Can you work these out from the model? Positions are in its coordinate system, mm. A direction names the side the tool comes from. Coordinates: 2 decimals unless noted, no trailing zeros. Order: outer loops, then holes, each group sorted by start corner. A loop starts at its lowest first (then second) coordinate and runs counter-clockwise, first axis right, second up.
```python
from build123d import *

# Parameters (mm, degrees)
F0_R           = 4.1275
F1_DEPTH       = 15.875
F3_D           = 8.255
F3_DEPTH       = 25.4
F3_CSINK_D     = 15.24
F3_CSINK_ANGLE = 90
F4_R           = 4.7625
F5_DEPTH       = 19.05


with BuildPart() as f1:
    # F0 (on Front) → F1 (new body)
    with BuildSketch(Plane.XZ):
        with BuildLine():
            ThreePointArc((0, -34.925), (-19.48747, -28.982653), (-32.343511, -13.177743))
            ThreePointArc((-32.343511, -13.177743), (-39.844625, -12.301191), (-45.625986, -17.160297))
            Line((-45.625986, -17.160297), (-72.23125, -70.2945))
            Line((-72.23125, -70.2945), (-72.23125, -89.3445))
            Line((-72.23125, -89.3445), (-56.35625, -89.3445))
            Line((-56.35625, -89.3445), (-56.35625, -86.1695))
            ThreePointArc((-56.35625, -86.1695), (-56.424398, -84.209267), (-56.35625, -82.249034))
            ThreePointArc((-56.35625, -82.249034), (-47.874791, -63.97181), (-29.36658, -56.007))
            ThreePointArc((-29.36658, -56.007), (-28.197928, -55.982797), (-27.029276, -56.007))
            Line((-27.029276, -56.007), (0, -56.007))
            Line((0, -56.007), (0, -34.925))
        make_face()
        with Locations((-37.109015, -21.4249)):
            Circle(F0_R, mode=Mode.SUBTRACT)
        with BuildLine():
            ThreePointArc((32.343511, -13.177743), (19.48747, -28.982653), (0, -34.925))
            Line((0, -34.925), (0, -56.007))
            Line((0, -56.007), (27.029276, -56.007))
            ThreePointArc((27.029276, -56.007), (28.197928, -55.982797), (29.36658, -56.007))
            ThreePointArc((29.36658, -56.007), (47.874791, -63.97181), (56.35625, -82.249034))
            ThreePointArc((56.35625, -82.249034), (56.424398, -84.209267), (56.35625, -86.1695))
            Line((56.35625, -86.1695), (56.35625, -89.3445))
            Line((56.35625, -89.3445), (72.23125, -89.3445))
            Line((72.23125, -89.3445), (72.23125, -70.2945))
            Line((72.23125, -70.2945), (45.625986, -17.160297))
            ThreePointArc((45.625986, -17.160297), (39.844625, -12.301191), (32.343511, -13.177743))
        make_face()
        with Locations((37.109015, -21.4249)):
            Circle(F0_R, mode=Mode.SUBTRACT)
        with BuildLine():
            Line((-29.36658, -56.007), (-27.029276, -56.007))
            ThreePointArc((-27.029276, -56.007), (-28.197928, -55.982797), (-29.36658, -56.007))
        make_face()
        with BuildLine():
            ThreePointArc((29.36658, -56.007), (28.197928, -55.982797), (27.029276, -56.007))
            Line((27.029276, -56.007), (29.36658, -56.007))
        make_face()
        with BuildLine():
            Line((-56.35625, -86.1695), (-56.35625, -82.249034))
            ThreePointArc((-56.35625, -82.249034), (-56.424398, -84.209267), (-56.35625, -86.1695))
        make_face()
        with BuildLine():
            ThreePointArc((56.35625, -86.1695), (56.424398, -84.209267), (56.35625, -82.249034))
            Line((56.35625, -82.249034), (56.35625, -86.1695))
        make_face()
    extrude(amount=F1_DEPTH)

    # F3
    with Locations(Plane.XZ.offset(15.875)):
        with Locations((-37.109015, -21.4249), (37.109015, -21.4249)):
            CounterSinkHole(F3_D / 2, F3_CSINK_D / 2, depth=F3_DEPTH, counter_sink_angle=F3_CSINK_ANGLE)

    # F4 (on face) → F5 (cut)
    with BuildSketch(Plane(origin=(0, 0, -89.3445), x_dir=(1, 0, 0), z_dir=(0, 0, -1))):
        with Locations((-64.5, 7.9375)):
            Circle(F4_R)
        with Locations((64.5, 7.9375)):
            Circle(F4_R)
    extrude(amount=-F5_DEPTH, mode=Mode.SUBTRACT)


solid = f1.part
```
1. Imagine slicing it at B-B on x = 64.5. Please give me the cut outline in (y, z) (1 decimal).
Completed:
outline: (-15.9, -89.3) - (-12.7, -89.3) - (-12.7, -70.3) - (-3.2, -70.3) - (-3.2, -89.3) - (0, -89.3) - (0, -54.9) - (-15.9, -54.9) - close
2. Imagine slicing it at A-A on y = -14.25. Give the number of separate pieces and of enclosed holes in the cut face, then the cut area to 3 significant figures.
Completed:
separate pieces: 1
enclosed holes: 2
area: 4,720 mm2
3. Please list where these lines run through material, in increasing order: probe 1 along Y at (x, z) = (-64.5, -82.75) (3 decimals); probe 2 along Z at (x, y) = (40, -14); probe 3 along Y at (x, z) = (61, -86) (3 decimals).
Completed:
probe 1: y = -15.875 to -12.7, -3.175 to 0
probe 2: z = -58.57 to -26.39, -16.46 to -12.35
probe 3: y = -15.875 to -11.167, -4.708 to 0
4. Imagine slicing it at C-C on x = -23. Please give me the cut outline in (y, z) (3 decimals), then the cut area to 3 significant figures.
Completed:
outline: (-15.875, -56.007) - (0, -56.007) - (0, -26.282) - (-15.875, -26.282) - close
area: 472 mm2
5. Thinking about a two-plate mould opening in X: for faces 1 (the flat face through (-72.231, -8, -80)), 2 (the cylindrical face through (-48.081, -7.826, -64.174)), 3 (the flat face through (72.231, -8, -80)), 4 (the flat face through (-1, 0, -50)), which applies, pulls with the +X half, pulls with the -X half, needs draft (parallel to the pull), parting line crosses it, or undercut?
Completed:
face 1: pulls with the -X half
face 2: undercut
face 3: pulls with the +X half
face 4: needs draft
6. I'm going to push flat-ended pins straight in: pin 1 (8 mm diameter, centred on x = 6.5, y = -8, fed in from -Z); pin 2 (5 mm diameter, centred on x = 64.5, y = -10, fed in from -Z); pin 3 (4 mm diameter, centred on x = 1, y = -14, fed in from +Z); pin 4 (5 mm diameter, centred on x = 35, z = -27.5, fed in from +Y). Where does each tip first touch, or does it pass through?
Completed:
pin 1: stops at z = -56.01
pin 2: stops at z = -70.29
pin 3: stops at z = -34.8
pin 4: stops at y = 0
7. On a 3-axis mill with a long thin cutter (end or side, diameter ignored), from which of +Z, -Z, +X, -X, +Y, -Y can I reach the whole of each face in a straight line? I mean faces 5 (the cylindrical face through (59.742, -8.147, -79.953)), 6 (the flat face through (0, -8, -56.007)), 7 (the flat face through (-68, -4, -89.344)). Say none if no direction works.
Completed:
face 5: -Z
face 6: -Z, +Y, -Y
face 7: -Z, +X, -X, +Y, -Y
